Source: CAD feature listing. Evaluate the final solid. Frame: model axes, mm. Face numbers are marked on the shaded views. Give positions to 0.01 mm unless a question says otherwise; leave off trailing zeros. Loops run counter-clockwise (first coordinate to the right, second up) from the corner with the lowest first, then second, coordinate; pieces in that order, holes last. Notation, with made-up numbers: M 66.5,53.25 L 91.5,53.25 A30 ccw 91.5,75.25 Z; hole C 66.5,-32 d11. An arc over 180 degrees is marked long. Write item = value, one per line.
from build123d import *

# Parameters (mm, degrees)
SKETCH1_W               = 89.5
SKETCH1_H               = 125
BOSS_EXTRUDE1_DEPTH     = 8
SKETCH2_R               = 7.5
SKETCH2_R_2             = 3
CUT_EXTRUDE1_DEPTH      = 4
SKETCH3_R               = 7.5
CUT_EXTRUDE2_DEPTH      = 154.789629039
SKETCH4_W               = 125
SKETCH4_H               = 22
SKETCH4_R               = 1.5
BOSS_EXTRUDE2_DEPTH     = 6
SKETCH5_R               = 1.5
CUT_EXTRUDE3_DEPTH      = 156.303734662
SKETCH8_W               = 125
SKETCH8_H               = 30
BOSS_EXTRUDE3_DEPTH     = 6
BOSS_EXTRUDE4_DEPTH     = 70
CUT_EXTRUDE5_DEPTH      = 217.645447679
CUT_EXTRUDE5_DEPTH_BACK = 217.645447679
SKETCH9_R               = 1.5
FILLET2_R               = 5
SKETCH12_R              = 1.5
CUT_EXTRUDE6_DEPTH      = 216.683216779


with BuildPart() as part:
    # Sketch1 → Boss-Extrude1 (new body)
    with BuildSketch(Plane(origin=(0, 0, 0), x_dir=(1, 0, 0), z_dir=(0, 1, 0))):
        with Locations((44.75, 62.5)):
            Rectangle(SKETCH1_W, SKETCH1_H)
    extrude(amount=BOSS_EXTRUDE1_DEPTH)

    # Sketch2 → Cut-Extrude1 (cut)
    with BuildSketch(Plane(origin=(0, 8, 0), x_dir=(-1, 0, 0), z_dir=(0, 1, 0))):
        with Locations(Location((-36.75, -90, 0), (0, 0, 90))):
            Circle(SKETCH2_R)
        with Locations(Location((-57.75, -90, 0), (0, 0, 90))):
            Circle(SKETCH2_R_2)
        with Locations(Location((-47.25, -71.813466521, 0), (0, 0, 90))):
            Circle(SKETCH2_R_2)
        with Locations(Location((-26.25, -71.813466521, 0), (0, 0, 90))):
            Circle(SKETCH2_R_2)
        with Locations(Location((-15.75, -90, 0), (0, 0, 90))):
            Circle(SKETCH2_R_2)
        with Locations(Location((-26.25, -108.186533479, 0), (0, 0, 90))):
            Circle(SKETCH2_R_2)
        with Locations(Location((-47.25, -108.186533479, 0), (0, 0, 90))):
            Circle(SKETCH2_R_2)
    extrude(amount=-CUT_EXTRUDE1_DEPTH, mode=Mode.SUBTRACT)

    # Sketch3 → Cut-Extrude2 (cut, through all)
    with BuildSketch(Plane(origin=(0, 4, 0), x_dir=(1, 0, 0), z_dir=(0, 1, 0))):
        with Locations(Location((36.75, 90, 0), (0, 0, 270))):
            Circle(SKETCH3_R)
    extrude(amount=-CUT_EXTRUDE2_DEPTH, mode=Mode.SUBTRACT)

    # Sketch4 → Boss-Extrude2 (add)
    with BuildSketch(Plane(origin=(89.5, 0, 0), x_dir=(0, 0, -1), z_dir=(1, 0, 0))):
        with Locations((62.5, 19)):
            Rectangle(SKETCH4_W, SKETCH4_H)
        with Locations((11.692170277, 24)):
            Circle(SKETCH4_R, mode=Mode.SUBTRACT)
        with Locations((36.692170277, 24)):
            Circle(SKETCH4_R, mode=Mode.SUBTRACT)
        with Locations((61.692170277, 24)):
            Circle(SKETCH4_R, mode=Mode.SUBTRACT)
        with Locations((86.692170277, 24)):
            Circle(SKETCH4_R, mode=Mode.SUBTRACT)
        with Locations((111.692170277, 24)):
            Circle(SKETCH4_R, mode=Mode.SUBTRACT)
    extrude(amount=-BOSS_EXTRUDE2_DEPTH)

    # Sketch5 → Cut-Extrude3 (cut, through all)
    with BuildSketch(Plane(origin=(0, 8, 0), x_dir=(-1, 0, 0), z_dir=(0, 1, 0))):
        with Locations(Location((-57.75, -90, 0), (0, 0, 90))):
            Circle(SKETCH5_R)
        with Locations(Location((-47.25, -71.813466521, 0), (0, 0, 90))):
            Circle(SKETCH5_R)
        with Locations(Location((-26.25, -71.813466521, 0), (0, 0, 90))):
            Circle(SKETCH5_R)
        with Locations(Location((-15.75, -90, 0), (0, 0, 90))):
            Circle(SKETCH5_R)
        with Locations(Location((-26.25, -108.186533479, 0), (0, 0, 90))):
            Circle(SKETCH5_R)
        with Locations(Location((-47.25, -108.186533479, 0), (0, 0, 90))):
            Circle(SKETCH5_R)
    extrude(amount=-CUT_EXTRUDE3_DEPTH, mode=Mode.SUBTRACT)

    # Sketch8 → Boss-Extrude3 (add)
    with BuildSketch(Plane.ZY):
        with Locations((-62.5, 15)):
            Rectangle(SKETCH8_W, SKETCH8_H)
    extrude(amount=BOSS_EXTRUDE3_DEPTH)

    # Sketch11 → Boss-Extrude4 (add)
    with BuildSketch(Plane(origin=(0, 0, -125), x_dir=(-1, 0, 0), z_dir=(0, 0, -1))):
        Polygon((6, 30), (0, 30), (0, 8), (-83.5, 8), (-83.5, 30), (-89.5, 30), (-89.5, 0), (6, 0), align=None)
    extrude(amount=BOSS_EXTRUDE4_DEPTH)

    # Sketch9 → Cut-Extrude5 (cut, two sides: drawn at the far end of the back side and taken through both)
    with BuildSketch(Plane(origin=(0, 0, 0), x_dir=(0, 0, -1), z_dir=(1, 0, 0)).offset(-CUT_EXTRUDE5_DEPTH_BACK)):
        with Locations((11.692170277, 24)):
            Circle(SKETCH9_R)
        with Locations((36.692170277, 24)):
            Circle(SKETCH9_R)
        with Locations((61.692170277, 24)):
            Circle(SKETCH9_R)
        with Locations((86.692170277, 24)):
            Circle(SKETCH9_R)
        with Locations((111.692170277, 24)):
            Circle(SKETCH9_R)
        with Locations(Location((136.692170277, 24, 0), (0, 0, 180))):
            Circle(SKETCH9_R)
        with Locations(Location((161.692170277, 24, 0), (0, 0, 180))):
            Circle(SKETCH9_R)
        with Locations(Location((186.692170277, 24, 0), (0, 0, 180))):
            Circle(SKETCH9_R)
    extrude(amount=CUT_EXTRUDE5_DEPTH + CUT_EXTRUDE5_DEPTH_BACK, mode=Mode.SUBTRACT)

    # Fillet2
    fillet2_edges = [part.edges().sort_by_distance(p)[0] for p in [
        (-6, 15, 0),
        (-6, 15, -195),
        (89.5, 15, -195),
        (89.5, 15, 0),
    ]]
    fillet(fillet2_edges, radius=FILLET2_R)

    # Sketch12 → Cut-Extrude6 (cut, through all)
    with BuildSketch(Plane(origin=(0, 8, 0), x_dir=(1, 0, 0), z_dir=(0, 1, 0))):
        with Locations(Location((41.75, 18.29, 0), (0, 0, 270))):
            Circle(SKETCH12_R)
        with Locations(Location((33.089745962, 23.29, 0), (0, 0, 270))):
            Circle(SKETCH12_R)
        with Locations(Location((33.089745962, 33.29, 0), (0, 0, 270))):
            Circle(SKETCH12_R)
        with Locations(Location((41.75, 38.29, 0), (0, 0, 270))):
            Circle(SKETCH12_R)
        with Locations(Location((50.410254038, 33.29, 0), (0, 0, 270))):
            Circle(SKETCH12_R)
        with Locations(Location((50.410254038, 23.29, 0), (0, 0, 270))):
            Circle(SKETCH12_R)
    extrude(amount=-CUT_EXTRUDE6_DEPTH, mode=Mode.SUBTRACT)


solid = part.part
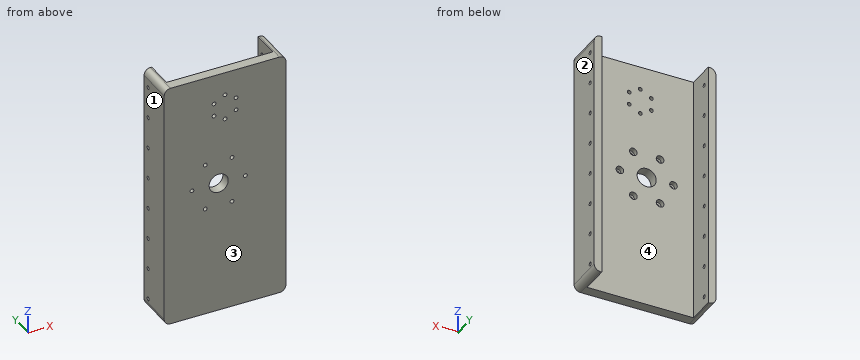
1. First-contact query: pin 1 Ø5 at (x, z) = (47.25, -108.19) entering from +Y; pin 2 Ø5 at (x, z) = (73.5, -70.5) entering from +Y. Flat tips, straight axial feed; report the tip coordinate or a pass-through.
Derived:
pin_1 = 4
pin_2 = 8
2. Cut plane A-A, the plane y = 18.5. Return the cut outline in (x, z).
Derived:
outline = M -6,-190 A5 ccw -1,-195 L 0,-195 L 0,0 L -1,0 A5 ccw -6,-5 Z; M 83.5,-195 L 84.5,-195 A5 ccw 89.5,-190 L 89.5,-5 A5 ccw 84.5,0 L 83.5,0 Z
3. Material intervals for probe 1 along X at (y, z) = (1.05, -90); probe 2 along Z at (x, y) = (50.5, 7.5); probe 3 along X at (y, z) = (17.25, -129.5), sorted ascending. Write a range as from..to.
Derived:
probe_1 = -6..14.25, 17.25..29.25, 44.25..56.25, 59.25..89.5
probe_2 = -195..-34.79, -31.79..-24.79, -21.79..0
probe_3 = -6..0, 83.5..89.5
4. Pull-direction query (X, two-part tool) for the marked faces 1, 2, 3 and 4; classes: +X half, -X half, draft (parallel to the pull), parting line (faces both ways), or undercut.
Derived:
face_1 = -X half
face_2 = +X half
face_3 = draft
face_4 = undercut
5. Cut plane C-C, the plane x = 6. Return the cut outline in (y, z), then the cut area to 3 significant figures.
Derived:
outline = M 0,-195 L 8,-195 L 8,0 L 0,0 Z
area = 1,560 mm²
6. Cut plane B-B, the plane z = -67. Return the cut outline in (x, y), then the cut area to 3 significant figures.
Derived:
outline = M -6,0 L 89.5,0 L 89.5,30 L 83.5,30 L 83.5,8 L 0,8 L 0,30 L -6,30 Z
area = 1,030 mm²
